from build123d import *

# Parameters (mm, degrees)
SKETCH1_R           = 14.2875
SKETCH1_R_2         = 1.524
SKETCH1_W           = 25.4
SKETCH1_H           = 5.08
BOSS_EXTRUDE1_DEPTH = 5.08
SKETCH2_W           = 5.08
SKETCH2_H           = 50.8
BOSS_EXTRUDE2_DEPTH = 5.08
SKETCH3_W           = 30.48
SKETCH3_H           = 5.08
CUT_EXTRUDE1_DEPTH  = 5.08


with BuildPart() as part:
    # Sketch1 → Boss-Extrude1 (new body)
    with BuildSketch(Plane.XY):
        Polygon((96.52, 198.12), (-96.52, 198.12), (-96.52, 0), (-66.04, 0), (-66.04, 5.08), (-35.56, 5.08), (-35.56, 0), (35.56, 0), (35.56, 5.08), (66.04, 5.08), (66.04, 0), (96.52, 0), align=None)
        Polygon((-62.23, 44.45), (-55.88, 44.45), (-49.53, 44.45), (-49.53, 41.275), (-62.23, 41.275), align=None, mode=Mode.SUBTRACT)
        with Locations((17.78, 27.94)):
            Circle(SKETCH1_R, mode=Mode.SUBTRACT)
        Polygon((62.23, 44.45), (68.58, 44.45), (74.93, 44.45), (74.93, 41.275), (62.23, 41.275), align=None, mode=Mode.SUBTRACT)
        with Locations((-50.8, 76.2)):
            Circle(SKETCH1_R_2, mode=Mode.SUBTRACT)
        with BuildLine():
            ThreePointArc((0, 74.676), (-1.077630735, 75.122369265), (-1.524, 76.2))
            ThreePointArc((-1.524, 76.2), (-1.077630735, 77.277630735), (0, 77.724))
            ThreePointArc((0, 77.724), (1.077630735, 77.277630735), (1.524, 76.2))
            ThreePointArc((1.524, 76.2), (1.077630735, 75.122369265), (0, 74.676))
        make_face(mode=Mode.SUBTRACT)
        with Locations((-50.8, 104.14)):
            Rectangle(SKETCH1_W, SKETCH1_H, mode=Mode.SUBTRACT)
        with Locations((50.8, 76.2)):
            Circle(SKETCH1_R_2, mode=Mode.SUBTRACT)
        with Locations((50.8, 104.14)):
            Rectangle(SKETCH1_W, SKETCH1_H, mode=Mode.SUBTRACT)
    extrude(amount=BOSS_EXTRUDE1_DEPTH)

    # Sketch2 → Boss-Extrude2 (add)
    with BuildSketch(Plane.XY.offset(5.08)):
        with Locations((99.06, 25.4)):
            Rectangle(SKETCH2_W, SKETCH2_H)
        with Locations((-99.06, 25.4)):
            Rectangle(SKETCH2_W, SKETCH2_H)
    extrude(amount=-BOSS_EXTRUDE2_DEPTH)

    # Sketch3 → Cut-Extrude1 (cut)
    with BuildSketch(Plane.XY.offset(5.08)):
        with Locations((0, 111.76)):
            Rectangle(SKETCH3_W, SKETCH3_H)
    extrude(amount=-CUT_EXTRUDE1_DEPTH, mode=Mode.SUBTRACT)


solid = part.part
Geometry: final body of the model. Coordinates: model frame, mm. A direction names the side the tool comes from. Round coordinates to 2 decimals unless told otherwise and drop trailing zeros. Write each loop counter-clockwise with the first axis right and the second up, starting at its lowest first coordinate (ties: lowest second). Pieces come first, ordered by that corner, then holes. Notation, with made-up numbers: M 66.5,-14.75 L 111.5,-14.75 A27 cw 111.5,21.25 Z; hole C -15.75,-16.5 d7. An arc over 180 degrees is marked long. Write item = value, one per line.
Item 1: Access query for faces 5 (the face through (-84, 0, 3)), 6 (the face through (-51, 106.68, 3)), 7 (the face through (66.04, 3, 3)), 8 (the face through (-96.52, 125, 3)). Directions: +Z, -Z, +X, -X, +Y, -Y. A direction counts if a zero-diameter tool reaches every point of the face in a straight line with its end or side. Return the directions, or none.
Findings:
face_5 = +Z, -Z, +X, -X, -Y
face_6 = +Z, -Z
face_7 = +Z, -Z, -Y
face_8 = +Z, -Z, -X, +Y
Item 2: Section query D-D on y = 70. Return loops of the section in (x, z), then the cut area to 3 significant figures.
Findings:
outline = M -96.52,0 L 96.52,0 L 96.52,5.08 L -96.52,5.08 Z
area = 981 mm^2
Item 3: Section query C-C on z = 2.05. State how many separate pieces and enclosed holes the cut face has, then the cut area to 3 significant figures.
Findings:
separate_pieces = 1
enclosed_holes = 9
area = 37,300 mm^2
Item 4: Pin query (flat end, axial travel): P1, Ø2.5, axis at y = 103.5, z = 4, coming from the +X side; P2, Ø2.5, axis at y = 104.5, z = 3, coming from the -X side; P3, Ø2.5, axis at x = 50.8, y = 76.2, coming from the -Z side. Return the tip coordinate at first contact, or that it passes through.
Findings:
P1 = 96.52
P2 = -96.52
P3 = through
Item 5: Pull-direction query (Y, two-part tool) for faces 1 (the face through (69, 41.275, 3)), 2 (the face through (-1, 100, 0)), 3 (the face through (51, 5.08, 3)), 4 (the face through (-15.24, 112, 3)); classes: pulls with the +Y half, pulls with the -Y half, needs draft (parallel to the pull), parting line crosses it, or undercut.
Findings:
face_1 = undercut
face_2 = needs draft
face_3 = pulls with the -Y half
face_4 = undercut
Item 6: Material intervals for line 1 along Y through (x, z) = (-50.8, 2.5) (3 decimals); line 2 along Y through (x, z) = (50.8, 2.8); line 3 along Y through (x, z) = (-57, 3.65) (3 decimals), sorted ascending. Write a range as [from, to].
Findings:
line_1 = [5.08, 41.275], [44.45, 74.676], [77.724, 101.6], [106.68, 198.12]
line_2 = [5.08, 74.68], [77.72, 101.6], [106.68, 198.12]
line_3 = [5.08, 41.275], [44.45, 101.6], [106.68, 198.12]
Item 7: Section query A-A on y = 27.94. Return loops of the section in (x, z).
Findings:
outline = M -101.6,0 L 3.49,0 L 3.49,5.08 L -101.6,5.08 Z; M 32.07,0 L 101.6,0 L 101.6,5.08 L 32.07,5.08 Z
Item 8: Section query B-B on x = 17.78. Return loops of the section in (y, z), then the cut area to 3 significant figures.
Findings:
outline = M 0,0 L 13.65,0 L 13.65,5.08 L 0,5.08 Z; M 42.23,0 L 198.12,0 L 198.12,5.08 L 42.23,5.08 Z
area = 861 mm^2
